Verification items for the finished model (mm, model axes). Face numbers are marked on the shaded views. A direction names the side the tool comes from. Round coordinates to 2 decimals unless told otherwise and drop trailing zeros. Loops run counter-clockwise (first coordinate to the right, second up) from the corner with the lowest first, then second, coordinate; pieces in that order, holes last. Notation, with made-up numbers: M 48,-32 L 106,-32 A28 cw 106,-3 Z; hole C -37.5,-37 d6. An arc over 180 degrees is marked long. Write item = value, one per line. Start each with the question number.
from build123d import *

# Parameters (mm, degrees)
SKETCH_1_R               = 50
EXTRUDE_18_DEPTH         = 13
EXTRUDE_18_2_DEPTH       = 13
SKETCH_1_28_W            = 300
SKETCH_1_28_H            = 100
EXTRUDE_21_DEPTH         = 15
SKETCH_1_30_R            = 5
EXTRUDE_22_DEPTH         = 70
SKETCH_1_31_R            = 50
CUT_EXTRUDE_2_DEPTH      = 41
EXTRUDE_23_DEPTH         = 18
EXTRUDE_23_DEPTH_BACK    = 1
SKETCH_1_32_R            = 50
SKETCH_1_33_R            = 6.5
CUT_EXTRUDE_3_DEPTH      = 242.8
CUT_EXTRUDE_5_DEPTH      = 130
CUT_EXTRUDE_5_DEPTH_BACK = 69
SKETCH_1_35_R            = 3.175
SKETCH_1_36_R            = 50
CUT_EXTRUDE_6_DEPTH      = 34
EXTRUDE_24_DEPTH         = 18
EXTRUDE_24_DEPTH_BACK    = 3
SKETCH_1_37_R            = 50
CUT_EXTRUDE_7_DEPTH      = 87
CUT_EXTRUDE_7_DEPTH_BACK = 98
SKETCH_1_41_R            = 3.175


with BuildPart() as part:
    # Sketch 1 → Extrude 18 (new body)
    with BuildSketch(Plane.XY):
        with Locations(Location((0, 50, 0), (0, 0, 180))):
            Circle(SKETCH_1_R)
    extrude(amount=EXTRUDE_18_DEPTH)



with BuildPart() as body_2:
    # Sketch 1 → Extrude 18 2 (new body)
    with BuildSketch(Plane.XY):
        with Locations(Location((-300, 50, 0), (0, 0, 180))):
            Circle(SKETCH_1_R)
    extrude(amount=EXTRUDE_18_2_DEPTH)


with BuildPart() as part_1:
    add(part.part)

    add(body_2.part)  # Extrude 21 merges body 2
    # Sketch 1_28 → Extrude 21 (add)
    with BuildSketch(Plane.XY):
        with Locations((-150, 50)):
            Rectangle(SKETCH_1_28_W, SKETCH_1_28_H)
    extrude(amount=EXTRUDE_21_DEPTH)

    # Sketch 1_30 → Extrude 22 (add)
    with BuildSketch(Plane.XY):
        with Locations((-150, 50)):
            Circle(SKETCH_1_30_R)
    extrude(amount=EXTRUDE_22_DEPTH)

    # Sketch 1_31 → Cut-Extrude 2 (cut)
    with BuildSketch(Plane.XY):
        with Locations((-300, 50)):
            Circle(SKETCH_1_31_R)
    extrude(amount=CUT_EXTRUDE_2_DEPTH, mode=Mode.SUBTRACT)

    # Sketch 1_32 → Extrude 23 (add, two sides: drawn at the far end of the back side and taken through both)
    with BuildSketch(Plane.XY.offset(-EXTRUDE_23_DEPTH_BACK)):
        with Locations((-300, 50)):
            Circle(SKETCH_1_32_R)
    extrude(amount=EXTRUDE_23_DEPTH + EXTRUDE_23_DEPTH_BACK)

    # Sketch 1_33 → Cut-Extrude 3 (cut)
    with BuildSketch(Plane.XY):
        with Locations(Location((0, 50, 0), (0, 0, 90))):
            Circle(SKETCH_1_33_R)
    extrude(amount=CUT_EXTRUDE_3_DEPTH, mode=Mode.SUBTRACT)

    # Sketch 1_35 → Cut-Extrude 5 (cut, two sides: drawn at the far end of the back side and taken through both)
    with BuildSketch(Plane.XY.offset(-CUT_EXTRUDE_5_DEPTH_BACK)):
        with Locations((-261.469660941, 50)):
            Circle(SKETCH_1_35_R)
    extrude(amount=CUT_EXTRUDE_5_DEPTH + CUT_EXTRUDE_5_DEPTH_BACK, mode=Mode.SUBTRACT)

    # Sketch 1_36 → Cut-Extrude 6 (cut)
    with BuildSketch(Plane.XY):
        with Locations((0, 50)):
            Circle(SKETCH_1_36_R)
    extrude(amount=CUT_EXTRUDE_6_DEPTH, mode=Mode.SUBTRACT)

    # Sketch 1_37 → Extrude 24 (add, two sides: drawn at the far end of the back side and taken through both)
    with BuildSketch(Plane.XY.offset(-EXTRUDE_24_DEPTH_BACK)):
        with Locations((0, 50)):
            Circle(SKETCH_1_37_R)
    extrude(amount=EXTRUDE_24_DEPTH + EXTRUDE_24_DEPTH_BACK)

    # Sketch 1_41 → Cut-Extrude 7 (cut, two sides: drawn at the far end of the back side and taken through both)
    with BuildSketch(Plane.XY.offset(-CUT_EXTRUDE_7_DEPTH_BACK)):
        with Locations((-272.75493597, 77.24506403)):
            Circle(SKETCH_1_41_R)
        with BuildLine():
            ThreePointArc((-296.825, 88.530339059), (-297.75493597, 90.77540309), (-300, 91.705339059))
            Line((-300, 91.705339059), (-300, 85.355339059))
            ThreePointArc((-300, 85.355339059), (-297.75493597, 86.285275029), (-296.825, 88.530339059))
        make_face()
        with BuildLine():
            Line((-300, 85.355339059), (-300, 91.705339059))
            ThreePointArc((-300, 91.705339059), (-303.175, 88.530339059), (-300, 85.355339059))
        make_face()
        with Locations((-327.24506403, 77.24506403)):
            Circle(SKETCH_1_41_R)
        with Locations((-338.530339059, 50)):
            Circle(SKETCH_1_41_R)
        with BuildLine():
            ThreePointArc((-325, 25), (-329.490128061, 25), (-329.490128061, 20.509871939))
            Line((-329.490128061, 20.509871939), (-325, 25))
        make_face()
        with BuildLine():
            Line((-325, 25), (-329.490128061, 20.509871939))
            ThreePointArc((-329.490128061, 20.509871939), (-326.030044133, 19.821618454), (-324.07006403, 22.75493597))
            ThreePointArc((-324.07006403, 22.75493597), (-324.311746515, 23.969955867), (-325, 25))
        make_face()
        with BuildLine():
            ThreePointArc((-300, 14.644660941), (-303.175, 11.469660941), (-300, 8.294660941))
            Line((-300, 8.294660941), (-300, 14.644660941))
        make_face()
        with BuildLine():
            Line((-300, 14.644660941), (-300, 8.294660941))
            ThreePointArc((-300, 8.294660941), (-297.75493597, 9.22459691), (-296.825, 11.469660941))
            ThreePointArc((-296.825, 11.469660941), (-297.75493597, 13.714724971), (-300, 14.644660941))
        make_face()
        with Locations((-272.75493597, 22.75493597)):
            Circle(SKETCH_1_41_R)
        with BuildLine():
            ThreePointArc((-264.644660941, 50), (-261.469660941, 46.825), (-258.294660941, 50))
            Line((-258.294660941, 50), (-264.644660941, 50))
        make_face()
        with BuildLine():
            Line((-264.644660941, 50), (-258.294660941, 50))
            ThreePointArc((-258.294660941, 50), (-261.469660941, 53.175), (-264.644660941, 50))
        make_face()
        with Locations((-27.24506403, 22.75493597)):
            Circle(SKETCH_1_41_R)
        with Locations((-38.530339059, 50)):
            Circle(SKETCH_1_41_R)
        with Locations((-27.24506403, 77.24506403)):
            Circle(SKETCH_1_41_R)
        with BuildLine():
            ThreePointArc((3.175, 88.530339059), (2.24506403, 90.77540309), (0, 91.705339059))
            Line((0, 91.705339059), (0, 85.355339059))
            ThreePointArc((0, 85.355339059), (2.24506403, 86.285275029), (3.175, 88.530339059))
        make_face()
        with BuildLine():
            Line((0, 85.355339059), (0, 91.705339059))
            ThreePointArc((0, 91.705339059), (-3.175, 88.530339059), (0, 85.355339059))
        make_face()
        with Locations((27.24506403, 77.24506403)):
            Circle(SKETCH_1_41_R)
        with Locations((27.24506403, 22.75493597)):
            Circle(SKETCH_1_41_R)
        with Locations((38.530339059, 50)):
            Circle(SKETCH_1_41_R)
        with BuildLine():
            ThreePointArc((0, 14.644660941), (-3.175, 11.469660941), (0, 8.294660941))
            Line((0, 8.294660941), (0, 14.644660941))
        make_face()
        with BuildLine():
            Line((0, 14.644660941), (0, 8.294660941))
            ThreePointArc((0, 8.294660941), (2.24506403, 9.22459691), (3.175, 11.469660941))
            ThreePointArc((3.175, 11.469660941), (2.24506403, 13.714724971), (0, 14.644660941))
        make_face()
    extrude(amount=CUT_EXTRUDE_7_DEPTH + CUT_EXTRUDE_7_DEPTH_BACK, mode=Mode.SUBTRACT)


solid = part_1.part
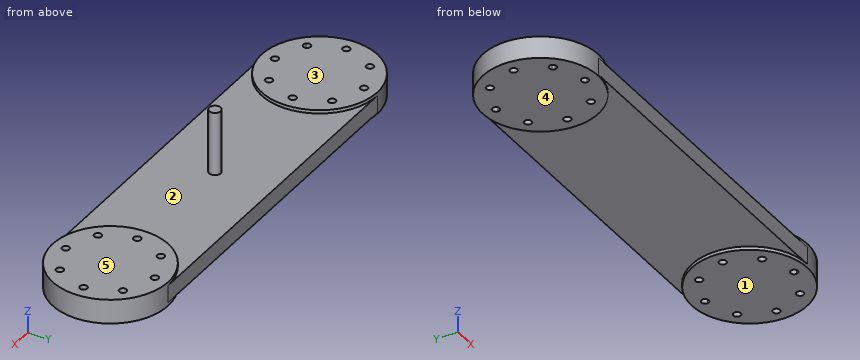
1. Section check C-C, the plane z = 38. Enter the section's corners in (x, y).
2. Tool access check on the marked faces 3, 4 and 5. Record the directions out of +Z, -Z, +X, -X, +Y, -Y that give a thin tool (end or side, any length) a straight path to the whole face; none if there is none.
3. Section check B-B, the plane y = 68. Enter the section's corners in (x, z), and give its area (3 significant figures).
4. Section check A-A, the plane x = -150. Enter the section's corners in (y, z), and give its area (3 significant figures).
5. Mould release check, pull along X, two halves, no side actions. Record for the marked faces 1 and 2: pulls with the +X half, pulls with the -X half, needs draft (parallel to the pull), parting line crosses it, or undercut.
6. Thickness scan on line 1 (Z direction, x = -255, y = 72); line 2 (Z direction, x = 32.5, y = 83); line 3 (X direction, y = 57, z = 16). Record the ranges inside material, lowest first.
7. Gauge pin test, flat ends, axial feed: P1, Ø8.5, axis at x = -338.53, y = 50, coming from the +Z side; P2, Ø5.5, axis at x = 27.25, y = 22.75, coming from the +Z side; P3, Ø8.5, axis at x = -27.25, y = 77.25, coming from the -Z side; P4, Ø8, axis at y = 57.5, z = 20.5, coming from the +X side. Record the tip position at first contact, or that the pin passes through.
Computed values:
q1.outline = C -150,50 d10
q2.face_3 = +Z, -X, +Y, -Y
q2.face_4 = -Z, -X, +Y, -Y
q2.face_5 = +Z, +X, +Y, -Y
q3.outline = M -346.65,-1 L -253.35,-1 L -253.35,0 L -46.65,0 L -46.65,-3 L 46.65,-3 L 46.65,18 L -46.65,18 L -46.65,15 L -253.35,15 L -253.35,18 L -346.65,18 Z
q3.area = 6,830 mm2
q4.outline = M 0,0 L 100,0 L 100,15 L 55,15 L 55,70 L 45,70 L 45,15 L 0,15 Z
q4.area = 2,050 mm2
q5.face_1 = needs draft
q5.face_2 = undercut
q6.line_1 = 0 to 15
q6.line_2 = -3 to 18
q6.line_3 = -349.51 to -250.49, -49.51 to 49.51
q7.P1 = 18
q7.P2 = through
q7.P3 = -3
q7.P4 = 49.81
